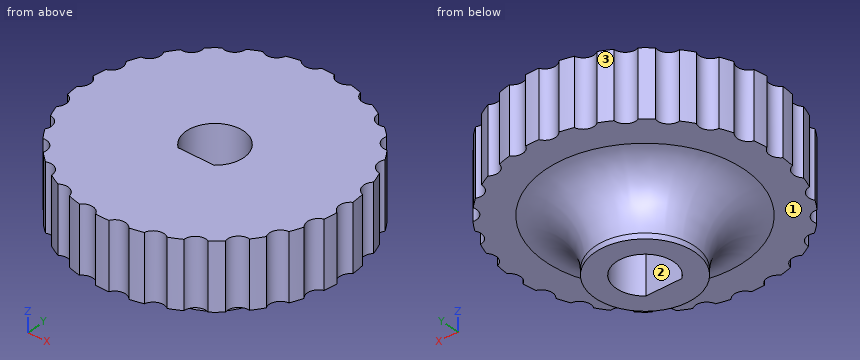
```python
from build123d import *

# Parameters (mm, degrees)
SKETCH019_R        = 4.5
PAD010_DEPTH       = 5
SKETCH020_R        = 12
PAD011_DEPTH       = 6
SKETCH021_R        = 1
POCKET006_DEPTH    = 6
POLARPATTERN_COUNT = 26
FILLET_R           = 4.5


with BuildPart() as part:
    # Sketch019 → Pad010 (new body)
    with BuildSketch(Plane(origin=(21.15, 21.15, 62.75), x_dir=(0, -1, 0), z_dir=(0, 0, 1))):
        Circle(SKETCH019_R)
        with BuildLine():
            ThreePointArc((2, 1.661325), (-2.6, 0), (2, -1.661325))
            Line((2, 1.661325), (2, -1.661325))
        make_face(mode=Mode.SUBTRACT)
    extrude(amount=PAD010_DEPTH)

    # Sketch020 → Pad011 (new body)
    with BuildSketch(Plane(origin=(21.15, 21.15, 67.75), x_dir=(0, -1, 0), z_dir=(0, 0, 1))):
        Circle(SKETCH020_R)
        with BuildLine():
            ThreePointArc((2, 1.661325), (-2.6, 0), (2, -1.661325))
            Line((2, 1.661325), (2, -1.661325))
        make_face(mode=Mode.SUBTRACT)
    extrude(amount=PAD011_DEPTH)

    # Sketch021 → Pocket006 (cut)
    with BuildSketch(Plane(origin=(21.15, 21.15, 73.75), x_dir=(0, -1, 0), z_dir=(0, 0, 1))):
        with Locations((0, 12.5)):
            Circle(SKETCH021_R)
    pocket006 = extrude(amount=-POCKET006_DEPTH, mode=Mode.SUBTRACT)

    # PolarPattern: Pocket006 ×26 about axis
    polarpattern_axis = Axis((21.15, 21.15, 73.75), (0, 0, 1))
    for i in range(1, POLARPATTERN_COUNT):
        add(pocket006.rotate(polarpattern_axis, i * 360 / POLARPATTERN_COUNT), mode=Mode.SUBTRACT)

    # Fillet
    fillet_edges = [part.edges().sort_by_distance(p)[0] for p in [
        (21.15, 25.65, 67.75),
    ]]
    fillet(fillet_edges, radius=FILLET_R)


solid = part.part
```
Input: part model. Units: mm. Frame: model coordinates. Face numbers are marked on the shaded views. A direction names the side the tool comes from. Give positions to 0.01 mm unless a question says otherwise; leave off trailing zeros. Write each loop counter-clockwise with the first axis right and the second up, starting at its lowest first coordinate (ties: lowest second). Pieces come first, ordered by that corner, then holes. Notation, with made-up numbers: (-15.5, -38) - (29.5, -38) arc R10 cw to (29.5, -24) - close; hole circle Ø3 at (2.5, 60.25). An arc over 180 degrees is marked (long way). Write item = value, one per line. Start each with the question number.
1. Section query B-B, the plane x = 21.15. Output: boundary loops of the cut face in (y, z).
2. Access query for the marked faces 1, 2 and 3. Directions: +Z, -Z, +X, -X, +Y, -Y. A direction counts if a zero-diameter tool reaches every point of the face in a straight line with its end or side. Return the directions, or none.
3. Ray query, L1, parallel to Y at x = 21.15, z = 71.75; L2, parallel to Z at x = 31.25, y = 23.5; L3, parallel to X at y = 21.15, z = 67. Return the intervals inside material, ascending.
4. First-contact query: pin 1 Ø1 at (x, z) = (30.5, 65.5) entering from -Y; pin 2 Ø1 at (y, z) = (25.5, 66) entering from -X; pin 3 Ø5 at (y, z) = (27, 64.5) entering from -X; pin 4 Ø3 at (x, z) = (23.5, 71) entering from +Y. Flat tips, straight axial feed; report the tip coordinate or a pass-through.
5. Section query C-C, the plane z = 65.25. Output: boundary loops of the cut face in (x, y).
6. Section query A-A, the plane y = 21.15. Output: boundary loops of the cut face in (x, z).
Check sheet entries:
q1.outline = (9.15, 67.75) - (12.15, 67.75) arc R4.5 cw to (16.65, 63.25) - (16.65, 62.75) - (19.15, 62.75) - (19.15, 73.75) - (9.15, 73.75) - close; (23.75, 62.75) - (25.65, 62.75) - (25.65, 63.25) arc R4.5 cw to (30.15, 67.75) - (33.15, 67.75) - (33.15, 73.75) - (23.75, 73.75) - close
q2.face_1 = -Z
q2.face_2 = +Z, -Z
q2.face_3 = +Z, -Z, -X, +Y
q3.L1 = 9.15 to 19.15, 23.75 to 33.15
q3.L2 = 67.75 to 73.75
q3.L3 = 14.64 to 18.55, 23.75 to 27.66
q4.pin_1 = through
q4.pin_2 = 17.02
q4.pin_3 = 17.18
q4.pin_4 = 32.93
q5.outline = circle Ø9.94 at (21.15, 21.15); hole (19.49, 19.15) - (22.81, 19.15) arc R2.6 ccw (long way) to start
q6.outline = (9.65, 67.75) - (12.15, 67.75) arc R4.5 cw to (16.65, 63.25) - (16.65, 62.75) - (18.55, 62.75) - (18.55, 73.75) - (9.65, 73.75) - close; (23.75, 62.75) - (25.65, 62.75) - (25.65, 63.25) arc R4.5 cw to (30.15, 67.75) - (32.65, 67.75) - (32.65, 73.75) - (23.75, 73.75) - close
